Verification items for the finished model (mm, model axes). A direction names the side the tool comes from. Round coordinates to 2 decimals unless told otherwise and drop trailing zeros. Write each loop counter-clockwise with the first axis right and the second up, starting at its lowest first coordinate (ties: lowest second). Pieces come first, ordered by that corner, then holes. Notation, with made-up numbers: (15.25, 31.25) -> (52.25, 31.25) arc R22 cw to (52.25, 68.25) -> close; hole circle Ø2 at (-19.75, -1). An arc over 180 degrees is marked (long way). Use CSV: the item, a comma, the result in double quotes.
Autodesk Fusion 360 part; units mm, degrees
sketch "Sketch1" plane through (0, 0, 0) normal (1, 0, 0) x (0, 0, -1)
  line L0 (0, 0) -> (0, 50.8)
  line L1 (0, 50.8) -> (6.35, 50.8)
  line L2 (6.35, 50.8) -> (6.35, 31.75)
  line L3 (6.35, 31.75) -> (9.525, 28.575)
  line L4 (9.525, 28.575) -> (34.1224, 28.575)
  line L5 (34.1224, 28.575) -> (35.9555, 25.4)
  line L6 (35.9555, 25.4) -> (39.1305, 25.4)
  line L7 (39.1305, 25.4) -> (40.9636, 28.575)
  line L8 (40.9636, 28.575) -> (44.1386, 28.575)
  line L9 (44.1386, 28.575) -> (45.9717, 25.4)
  line L10 (45.9717, 25.4) -> (49.1467, 25.4)
  line L11 (49.1467, 25.4) -> (50.9798, 28.575)
  line L12 (50.9798, 28.575) -> (54.1548, 28.575)
  line L13 (54.1548, 28.575) -> (58.7375, 20.6375)
  line L14 (58.7375, 20.6375) -> (63.5, 20.6375)
  line L15 (63.5, 20.6375) -> (63.5, 25.4)
  line L16 (63.5, 25.4) -> (88.9, 25.4)
  line L17 (88.9, 25.4) -> (88.9, 15.875)
  line L18 (88.9, 15.875) -> (85.725, 15.875)
  line L19 (85.725, 15.875) -> (85.725, 17.4625)
  line L20 (85.725, 17.4625) -> (82.55, 17.4625)
  line L21 (82.55, 17.4625) -> (82.55, 15.875)
  line L22 (82.55, 15.875) -> (76.2, 15.875)
  line L23 (76.2, 15.875) -> (76.2, 12.7)
  line L24 (76.2, 12.7) -> (63.5, 12.7)
  line L25 (63.5, 12.7) -> (63.5, 0)
  line L26 (63.5, 0) -> (12.7, 0)
  line L27 (12.7, 0) -> (12.7, 12.7)
  line L28 (12.7, 12.7) -> (6.35, 12.7)
  line L29 (6.35, 12.7) -> (6.35, 15.875)
  line L30 (6.35, 15.875) -> (0, 15.875)
  dimension "d1" = 6.35
  dimension "d2" = 45
  dimension "d3" = 3.175
  dimension "d4" = 57.15
  dimension "d5" = 3.175
  dimension "d6" = 60
  dimension "d7" = 60
  dimension "d8" = 60
  dimension "d9" = 60
  dimension "d10" = 60
  dimension "d11" = 4.7625
  dimension "d12" = 50.8
  dimension "d13" = 12.7
  dimension "d14" = 25.4
  dimension "d15" = 31.75
  dimension "d16" = 6.35
  dimension "d17" = 3.175
  dimension "d18" = 3.175
  dimension "d19" = 34.925
  dimension "d20" = 88.9
  dimension "d21" = 25.4
  dimension "d22" = 12.7
  dimension "d23" = 25.4
  dimension "d24" = 41.275
  dimension "d25" = 3.175
  dimension "d26" = 101.6
revolve "Revolve1" add sketch "Sketch1" angle 360 about axis through (0, 0, -63.5) along (0, 0, 1)
chamfer "Chamfer1" distance 1.5875 angle 45 3 edges at (-23.6811, 9.185, -63.5) (-23.6811, 9.185, -88.9) (-14.8007, 5.7406, -88.9)
thread "Thread1"
sketch "Sketch2" plane through (0, 0, 0) normal (0, 0, 1) x (1, 0, 0)
  circle A0 centre (0, 0) radius 15.875
  circle A1 centre (0, 0) radius 50.8
  circle A2 centre (0, 44.45) radius 3.175
  dimension "d29" = 44.45
  dimension "d30" = 6.35
extrude "Extrude1" cut sketch "Sketch2" against normal through all contours A2
pattern_circular "C-Pattern1" count 10 over 360 about axis through (0, 0, 0) along (0, 0, -1) of "Extrude1"
equation "d7 = d6"
equation "d8 = d6"
equation "d9 = d6"
equation "d10 = d6"
Q1. Section check B-B (x = 0). State how many separate pieces and enclosed holes the cut face has, plus the area to 3 significant figures.
Filled in:
separate pieces,"3"
enclosed holes,"0"
area,"3,850 mm²"
Q2. Section check A-A (y = 44.45). Record the cut outline in (x, z) (3 decimals).
Filled in:
outline,"(-24.593, -6.35) -> (-3.175, -6.35) -> (-3.175, 0) -> (-24.593, 0) -> close; (3.175, -6.35) -> (24.593, -6.35) -> (24.593, 0) -> (3.175, 0) -> close"
Q3. Section check C-C (z = -74). Record the cut outline in (x, y).
Filled in:
outline,"circle Ø50.8 at (0, 0); hole circle Ø25.4 at (0, 0)"
Q4. Material ranges on L1, parallel to Y at x = 0, z = -4.25 (3 decimals); L2, parallel to X at y = 0, z = -78 (3 decimals); L3, parallel to Y at x = 0, z = -70.75, recorded low to high.
Filled in:
L1,"-50.8 to -47.625, -41.275 to -15.875, 15.875 to 41.275, 47.625 to 50.8"
L2,"-25.4 to -15.875, 15.875 to 25.4"
L3,"-25.4 to -12.7, 12.7 to 25.4"
Q5. Go/stop test with flat-tipped pins: P1, Ø23, axis at x = 0, y = 0, coming from the +Z side; P2, Ø5, axis at x = 26.13, y = 35.96, coming from the +Z side; P3, Ø1, axis at x = 13, y = 22.5, coming from the -Z side; P4, Ø4, axis at x = -4, z = -41.5, coming from the +Y side. Record where each tip stops, or that it passes through.
Filled in:
P1,"z = -12.7"
P2,"through"
P3,"z = -55.94"
P4,"y = 28.5"
Q6. Mould release check, pull along Z, two halves, no side actions. Record for faces 6 (the conical face through (25.381, -3.332, -39.245)), 7 (the flat face through (0, 0, -12.7)), 8 (the cylindrical face through (1.256, -28.547, -21.996)): released by +Z, released by -Z, zero draft, split by the parting line, or undercut.
Filled in:
face 6,"undercut"
face 7,"released by +Z"
face 8,"zero draft"
Q7. Access from +Z, -Z, +X, -X, +Y, -Y to the whole of each face (thin tool, end or side, straight path). Record for faces 1 (the flat face through (-11, -7, -6.35)), 2 (the cylindrical face through (25.66, 32.82, -3.13)), 3 (the flat face through (-20, -7, -63.5)), 4 (the flat face through (0, 0, -63.5)), 5 (the flat face through (-12.5, -12.5, -88.9)).
Filled in:
face 1,"+Z"
face 2,"+Z, -Z"
face 3,"none"
face 4,"-Z"
face 5,"-Z, +X, -X, +Y, -Y"
Q8. Section check D-D (z = -27.5). Record the cut outline in (x, y) (3 decimals), plus the area to 3 significant figures.
Filled in:
outline,"circle Ø57.15 at (0, 0)"
area,"2,570 mm²"
